```python
from build123d import *

# Parameters (mm, degrees)
SKETCH_1_W          = 6.01304928
SKETCH_1_H          = 10
SKETCH_1_R          = 1.5
EXTRUDE_1_DEPTH     = 54
EXTRUDE_2_DEPTH     = 54
SKETCH_3_W          = 11.000516989
SKETCH_3_H          = 44
CUT_EXTRUDE_1_DEPTH = 54
FILLET_1_R          = 3
SKETCH_4_R          = 1.5
CUT_EXTRUDE_2_DEPTH = 65.758340749
CUT_EXTRUDE_START   = -8
SKETCH_5_R          = 1.5
CUT_EXTRUDE_3_DEPTH = 8
CUT_EXTRUDE_START_2 = -2.5
SKETCH_6_R          = 3.25
SKETCH_6_R_2        = 1.5
CUT_EXTRUDE_4_DEPTH = 2.5
FILLET_2_R          = 8


with BuildPart() as part:
    # 草图1 → 凸台-拉伸1 (new body)
    with BuildSketch(Plane.XY):
        Rectangle(SKETCH_1_W, SKETCH_1_H)
        Circle(SKETCH_1_R, mode=Mode.SUBTRACT)
    extrude(amount=EXTRUDE_1_DEPTH)

    # 草图2 → 凸台-拉伸2 (add)
    with BuildSketch(Plane.XY.offset(54)):
        Polygon((-3.00652464, 4.869160707), (-5.333618016, 2.309357993), (-11.387673162, -4.350102667), (-19.506532138, -13.280847541), (-0.740319183, -30.341041136), (9.164728063, -19.445489164), (3.00652464, 5), (3.00652464, -5), (-3.00652464, -5), align=None)
    extrude(amount=-EXTRUDE_2_DEPTH)

    # 草图3 → 切除-拉伸1 (cut)
    with BuildSketch(Plane(origin=(-15.436861734, -16.980547908, 0), x_dir=(0.7399400733959437, -0.6726727939963125, 0), z_dir=(-0.6726727939963125, -0.7399400733959437, 0))):
        with Locations((9.361542588, 27)):
            Rectangle(SKETCH_3_W, SKETCH_3_H)
    extrude(amount=-CUT_EXTRUDE_1_DEPTH, mode=Mode.SUBTRACT)

    # 圆角1
    fillet_1_edges = [part.edges().sort_by_distance(p)[0] for p in [
        (-19.506532138, -13.280847541, 27),
        (4.21220444, -24.89326515, 54),
        (9.164728063, -19.445489164, 27),
        (-10.123425661, -21.810944338, 54),
        (-0.740319183, -30.341041136, 27),
        (4.21220444, -24.89326515, 0),
        (-10.123425661, -21.810944338, 0),
        (1.629252849, -20.301477526, 5),
        (-4.053507722, -10.199069972, 5),
        (-4.053507722, -10.199069972, 49),
        (1.629252849, -20.301477526, 49),
    ]]
    fillet(fillet_1_edges, radius=FILLET_1_R)

    # 草图4 → 切除-拉伸2 (cut, through all)
    with BuildSketch(Plane(origin=(-4.069670404, 3.699700367, 0), x_dir=(0, 0, 1), z_dir=(-0.7399400733959431, 0.6726727939963131, 0))):
        with Locations(Location((22, -16.948544778, 0), (0, 0, 270))):
            Circle(SKETCH_4_R)
        with Locations(Location((32, -16.948544778, 0), (0, 0, 270))):
            Circle(SKETCH_4_R)
    extrude(amount=-CUT_EXTRUDE_2_DEPTH, mode=Mode.SUBTRACT)

    # 草图5 → 切除-拉伸3 (cut)
    # profile 1 of 3: a face of its own
    with BuildSketch(Plane(origin=(14.696542551, -13.360493228, 0), x_dir=(0, 0, -1), z_dir=(0.7399400733959434, -0.6726727939963129, 0)).offset(CUT_EXTRUDE_START)):
        with BuildLine():
            Line((-33.5, -19.948544778), (-30.5, -19.948544778))
            ThreePointArc((-30.5, -19.948544778), (-27.5, -16.948544778), (-30.5, -13.948544778))
            Line((-30.5, -13.948544778), (-33.5, -13.948544778))
            ThreePointArc((-33.5, -13.948544778), (-36.5, -16.948544778), (-33.5, -19.948544778))
        make_face()
        with Locations(Location((-32, -16.948544778, 0), (0, 0, 270))):
            Circle(SKETCH_5_R, mode=Mode.SUBTRACT)
    # profile 2 of 3: a face of its own
    with BuildSketch(Plane(origin=(14.696542551, -13.360493228, 0), x_dir=(0, 0, -1), z_dir=(0.7399400733959434, -0.6726727939963129, 0)).offset(CUT_EXTRUDE_START)):
        with BuildLine():
            ThreePointArc((-23.5, -13.948544778), (-26.5, -16.948544778), (-23.5, -19.948544778))
            Line((-23.5, -19.948544778), (-30.5, -19.948544778))
            ThreePointArc((-30.5, -19.948544778), (-27.5, -16.948544778), (-30.5, -13.948544778))
            Line((-30.5, -13.948544778), (-23.5, -13.948544778))
        make_face()
    # profile 3 of 3: a face of its own
    with BuildSketch(Plane(origin=(14.696542551, -13.360493228, 0), x_dir=(0, 0, -1), z_dir=(0.7399400733959434, -0.6726727939963129, 0)).offset(CUT_EXTRUDE_START)):
        with BuildLine():
            Line((-23.5, -19.948544778), (-20.5, -19.948544778))
            ThreePointArc((-20.5, -19.948544778), (-17.5, -16.948544778), (-20.5, -13.948544778))
            Line((-20.5, -13.948544778), (-23.5, -13.948544778))
            ThreePointArc((-23.5, -13.948544778), (-26.5, -16.948544778), (-23.5, -19.948544778))
        make_face()
        with Locations(Location((-22, -16.948544778, 0), (0, 0, 270))):
            Circle(SKETCH_5_R, mode=Mode.SUBTRACT)
    extrude(amount=CUT_EXTRUDE_3_DEPTH, mode=Mode.SUBTRACT)

    # 草图6 → 切除-拉伸4 (cut)
    # profile 1 of 2: a face of its own
    with BuildSketch(Plane(origin=(2.857118835, -2.597380759, 0), x_dir=(0, 0, -1), z_dir=(0.7399400733959437, -0.6726727939963125, 0)).offset(CUT_EXTRUDE_START_2)):
        with Locations(Location((-32, -16.948544778, 0), (0, 0, 90))):
            Circle(SKETCH_6_R)
        with Locations(Location((-32, -16.948544778, 0), (0, 0, 270))):
            Circle(SKETCH_6_R_2, mode=Mode.SUBTRACT)
    # profile 2 of 2: a face of its own
    with BuildSketch(Plane(origin=(2.857118835, -2.597380759, 0), x_dir=(0, 0, -1), z_dir=(0.7399400733959437, -0.6726727939963125, 0)).offset(CUT_EXTRUDE_START_2)):
        with Locations(Location((-22, -16.948544778, 0), (0, 0, 90))):
            Circle(SKETCH_6_R)
        with Locations(Location((-22, -16.948544778, 0), (0, 0, 270))):
            Circle(SKETCH_6_R_2, mode=Mode.SUBTRACT)
    extrude(amount=CUT_EXTRUDE_4_DEPTH, mode=Mode.SUBTRACT)

    # 圆角2
    # the kernel refuses this fillet: 8 mm, written as the material it takes off along each edge
    with BuildSketch(Plane(origin=(3.00652464, 5, -15.578572112), x_dir=(0.24428365244033365, -0.9697038192924736, 0), z_dir=(0, 0, 1))) as fillet_2_piece_1:
        with BuildLine():
            CenterArc((6.231428845, -8), FILLET_2_R, 90, 74.267861836)
            Line((-1.468889641, -5.830876853), (-1.62289601, -5.78749439))
            ThreePointArc((-1.62289601, -5.78749439), (-0.889597431, -2.876353042), (-0.155152611, 0.039085384))
            Line((-0.155152611, 0.039085384), (0, 0.16))
            Line((0, 0.16), (6.231428845, 0.16))
            Line((6.231428845, 0.16), (6.231428845, 0))
        make_face()
    extrude(amount=85.157144223, mode=Mode.SUBTRACT)


solid = part.part
```
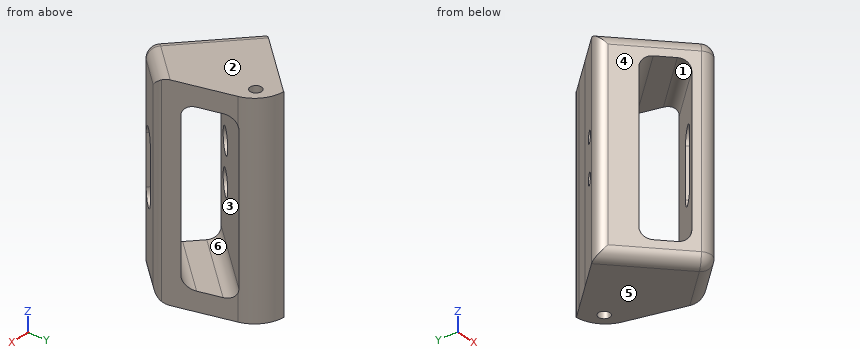
Geometry check sheet. Reference: the model listing, model coordinates, mm. Face numbers are marked on the shaded views. A direction names the side the tool comes from. Round coordinates to 2 decimals unless told otherwise and drop trailing zeros. Order: outer loops, then holes, each group sorted by start corner. A loop starts at its lowest first (then second) coordinate and runs counter-clockwise, first axis right, second up. Notation, with made-up numbers: (61, -20) - (92, -20) arc R15 ccw to (92, 6) - close; hole circle Ø11 at (20, 41.25). An arc over 180 degrees is marked (long way). Use a Markdown table: item, result. Add a question column.
(1) Release check for a two-part mould opening along Z. For the marked faces 1, 2, 3 and 4 record: pulls with the +Z half, pulls with the -Z half, needs draft (parallel to the pull), parting line crosses it, or undercut.
(2) Sectioned sample at A-A, the plane z = 42.5. Enter the section's corners in (x, y).
(3) Sectioned sample at B-B, the plane y = 0. Enter the section's corners in (x, z).
(4) Sectioned sample at C-C, the plane x = 0. Count the separate pieces of the cut face and the enclosed holes in it, and give its area (3 significant figures).
(5) Tool access check on the marked faces 5 and 6. Record the directions out of +Z, -Z, +X, -X, +Y, -Y that give a thin tool (end or side, any length) a straight path to the whole face; none if there is none.
(6) Material ranges on line 1 along Z through (x, y) = (-7.5, -19); line 2 along Z through (x, y) = (-8.75, -13.5); line 3 along Z through (x, y) = (-12.5, -13), recorded low to high. Write a range as [from, to].
(7) Depth check by flat-ended pin: pin 1 (4 mm diameter, centred on x = -12, z = 43, fed in from -Y); pin 2 (12 mm diameter, centred on y = -0.5, z = 37.5, fed in from -X). Enter the tip coordinate at first touch or a pass-through.
Answers below:
| question | item | result |
|---|---|---|
| 1 | face 1 | undercut |
| 1 | face 2 | pulls with the +Z half |
| 1 | face 3 | undercut |
| 1 | face 4 | needs draft |
| 2 | outline | (-17.49, -11.06) arc R3 ccw to (-17.29, -15.3) - (-12.58, -19.58) - (4.47, -0.82) arc R8 ccw to (-3.01, 5) - (-3.01, 4.87) - close; (-4.44, -26.98) - (-2.96, -28.32) arc R3 ccw to (1.28, -28.12) - (8.08, -20.64) arc R3 ccw to (8.77, -17.89) - (7.7, -13.63) - close; hole circle Ø3 at (0, 0) |
| 3 | outline | (-7.43, 0) - (-1.5, 0) - (-1.5, 54) - (-7.43, 54) - close; (1.5, 0) - (4.19, 0) - (4.19, 54) - (1.5, 54) - close |
| 4 | separate pieces | 2 |
| 4 | enclosed holes | 1 |
| 4 | area | 835 mm² |
| 5 | face 5 | -Z, +X, -X, +Y, -Y |
| 5 | face 6 | none |
| 6 | line 1 | [0, 5], [49, 54] |
| 6 | line 2 | [0, 18.93], [25.07, 28.93], [35.07, 54] |
| 6 | line 3 | [0, 20.96], [23.04, 30.96], [33.04, 54] |
| 7 | pin 1 | y = -19.58 |
| 7 | pin 2 | x = -13.34 |
